Verification items for this drawing (mm, ordinates from the low corner). Round coordinates to 2 decimals unless told otherwise and drop trailing zeros. Write each loop counter-clockwise with the first axis right and the second up, starting at its lowest first coordinate (ties: lowest second). Pieces come first, ordered by that corner, then holes.
Item 1: Depth check by flat-ended pin: P1, Ø7, axis at x = 7.5, z = 25, coming from the -Y side. Enter the tip coordinate at first touch or a pass-through.
Item 2: Scan lines: probe 1 along Z at (x, y) = (7.5, 2); probe 2 along X at (y, z) = (1.4, 25); probe 3 along X at (y, z) = (2.3, 27). Record each from-to range of solid material in increasing order.
Item 3: Cross-section at C-C (y = 1.3). Enter the section's corners in (x, z), then the cut area to 3 significant figures.
Item 4: Cross-section at B-B (z = 29). Enter the section's corners in (x, y), then the cut area to 3 significant figures.
Item 5: Cross-section at A-A (x = 9.5). Enter the section's corners in (y, z).
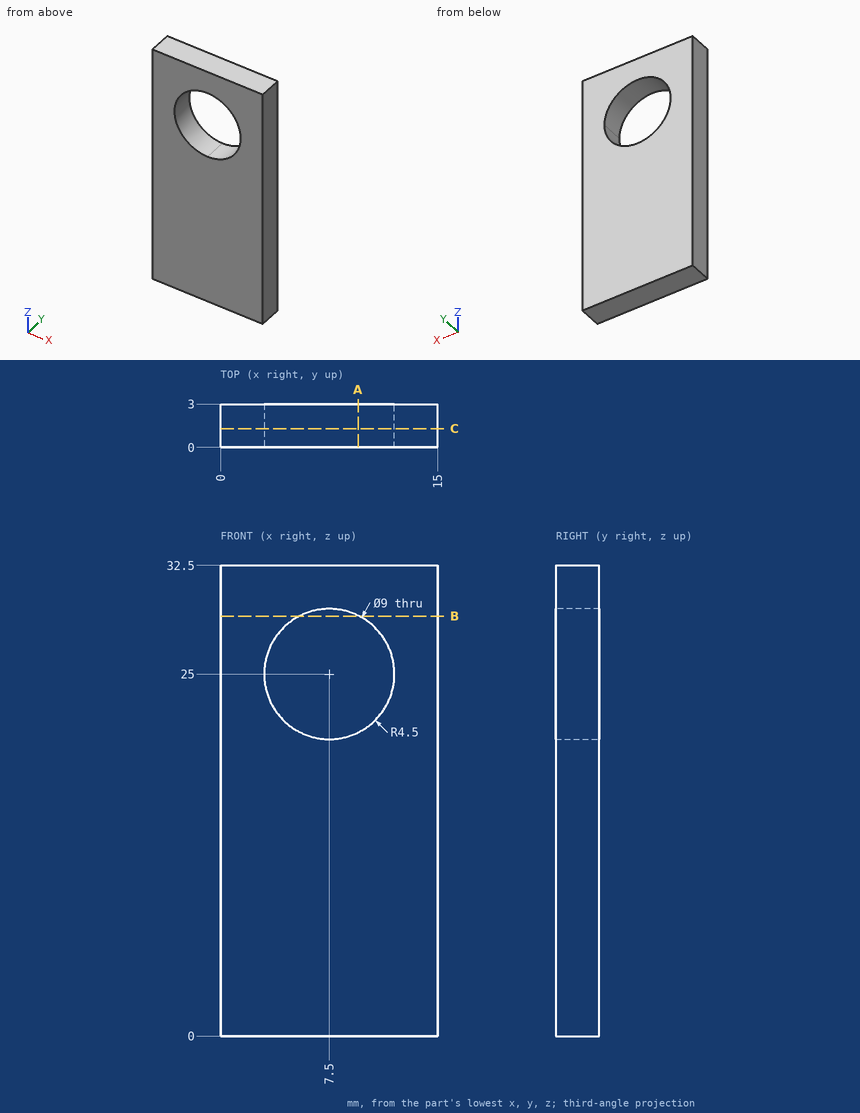
Resolved:
1. P1: passes through
2. probe 1: z = 0 to 20.5, 29.5 to 32.5
2. probe 2: x = 0 to 3, 12 to 15
2. probe 3: x = 0 to 3.47, 11.53 to 15
3. outline: (0, 0) - (15, 0) - (15, 32.5) - (0, 32.5) - close; hole circle Ø9 at (7.5, 25)
3. area: 424 mm2
4. outline: (0, 0) - (5.44, 0) - (5.44, 3) - (0, 3) - close; (9.56, 0) - (15, 0) - (15, 3) - (9.56, 3) - close
4. area: 32.6 mm2
5. outline: (0, 0) - (3, 0) - (3, 20.97) - (0, 20.97) - close; (0, 29.03) - (3, 29.03) - (3, 32.5) - (0, 32.5) - close
